For this review, take the finished solid that the model builds, in its own axes (mm). A direction names the side the tool comes from. Give positions to 0.01 mm unless a question says otherwise; leave off trailing zeros. Write item = value, one per line.
```python
from build123d import *

# Parameters (mm, degrees)
SKETCH1_R                 = 63.5
EXTRUDE1_DEPTH            = 6.35
SKETCH2_R                 = 58.7375
SKETCH2_R_2               = 52.3875
EXTRUDE2_DEPTH            = 12.7
SKETCH3_W                 = 1.5875
SKETCH3_H                 = 2.38125
CHAMFER1_SIZE             = 0.5
EXTRUDE3_DEPTH            = 6.35
F_6_CLEARANCE_HOLE1_D     = 3.7973
F_6_CLEARANCE_HOLE1_DEPTH = 330.2
F_6_CLEARANCE_HOLE1_TIP   = 1.140824014
FILLET1_R                 = 6.35
F_6_CLEARANCE_HOLE2_D     = 3.7973
F_6_CLEARANCE_HOLE2_DEPTH = 25.4
F_6_CLEARANCE_HOLE2_TIP   = 1.140824014
SKETCH8_R                 = 52.3875
CUT_EXTRUDE1_DEPTH        = 3.175


with BuildPart() as part:
    # Sketch1 → Extrude1 (new body)
    with BuildSketch(Plane(origin=(0, 0, 0), x_dir=(1, 0, 0), z_dir=(0, 1, 0))):
        Circle(SKETCH1_R)
    extrude(amount=EXTRUDE1_DEPTH)

    # Sketch2 → Extrude2 (add)
    with BuildSketch(Plane(origin=(0, 6.35, 0), x_dir=(-1, 0, 0), z_dir=(0, 1, 0))):
        Circle(SKETCH2_R)
        Circle(SKETCH2_R_2, mode=Mode.SUBTRACT)
    extrude(amount=EXTRUDE2_DEPTH)

    # Sketch3 → Cut-Revolve1 (revolve, cut)
    with BuildSketch(Plane(origin=(0, 0, 0), x_dir=(0, 0, -1), z_dir=(1, 0, 0))):
        with Locations((-57.94375, 15.656558664)):
            Rectangle(SKETCH3_W, SKETCH3_H)
        with Locations((-57.94375, 10.842416167)):
            Rectangle(SKETCH3_W, SKETCH3_H)
    revolve(axis=Axis((0, 0, 0), (0, 1, 0)), mode=Mode.SUBTRACT)

    # Chamfer1
    chamfer1_edges = [part.edges().sort_by_distance(p)[0] for p in [
        (58.7375, 16.847183664, 0),
        (58.7375, 14.465933664, 0),
        (58.7375, 12.033041167, 0),
        (58.7375, 9.651791167, 0),
        (58.7375, 19.05, 0),
        (52.3875, 19.05, 0),
    ]]
    chamfer(chamfer1_edges, length=CHAMFER1_SIZE)

    # Sketch5 → Extrude3 (add)
    with BuildSketch(Plane.XZ):
        with BuildLine():
            Line((-69.85, 9.525), (69.85, 9.525))
            ThreePointArc((69.85, 9.525), (74.340128061, 7.665128061), (76.2, 3.175))
            Line((76.2, 3.175), (76.2, -3.175))
            ThreePointArc((76.2, -3.175), (74.340128061, -7.665128061), (69.85, -9.525))
            Line((69.85, -9.525), (-69.85, -9.525))
            ThreePointArc((-69.85, -9.525), (-74.340128061, -7.665128061), (-76.2, -3.175))
            Line((-76.2, -3.175), (-76.2, 3.175))
            ThreePointArc((-76.2, 3.175), (-74.340128061, 7.665128061), (-69.85, 9.525))
        make_face()
    extrude(amount=-EXTRUDE3_DEPTH)

    # #6 Clearance Hole1
    with Locations(Plane(origin=(-69.85, 0, 0), x_dir=(0, 0, -1), z_dir=(0, -1, 0))):
        with Locations((0, 0), (0, 139.7)):
            Hole(F_6_CLEARANCE_HOLE1_D / 2, depth=F_6_CLEARANCE_HOLE1_DEPTH)
            with Locations((0, 0, -(F_6_CLEARANCE_HOLE1_DEPTH + F_6_CLEARANCE_HOLE1_TIP / 2))):  # 118° drill point
                Cone(0, F_6_CLEARANCE_HOLE1_D / 2, F_6_CLEARANCE_HOLE1_TIP, mode=Mode.SUBTRACT)

    # Fillet1
    fillet1_edges = [part.edges().sort_by_distance(p)[0] for p in [
        (62.781560788, 3.175, -9.525),
        (-62.781560788, 3.175, -9.525),
        (-62.781560788, 3.175, 9.525),
        (62.781560788, 3.175, 9.525),
    ]]
    fillet(fillet1_edges, radius=FILLET1_R)

    # #6 Clearance Hole2
    with Locations(Plane(origin=(25.4, 0, 19.05), x_dir=(0, 0, -1), z_dir=(0, -1, 0))):
        with Locations((0, 0), (-19.05, 0), (-19.05, -50.8), (0, -50.8)):
            Hole(F_6_CLEARANCE_HOLE2_D / 2, depth=F_6_CLEARANCE_HOLE2_DEPTH)
            with Locations((0, 0, -(F_6_CLEARANCE_HOLE2_DEPTH + F_6_CLEARANCE_HOLE2_TIP / 2))):  # 118° drill point
                Cone(0, F_6_CLEARANCE_HOLE2_D / 2, F_6_CLEARANCE_HOLE2_TIP, mode=Mode.SUBTRACT)

    # Sketch8 → Cut-Extrude1 (cut)
    with BuildSketch(Plane(origin=(0, 6.35, 0), x_dir=(-1, 0, 0), z_dir=(0, 1, 0))):
        Circle(SKETCH8_R)
    extrude(amount=-CUT_EXTRUDE1_DEPTH, mode=Mode.SUBTRACT)


solid = part.part
```
(1) To check wall thickness, follow probe 1 along X at (y, z) = (3.25, 0); probe 2 along X at (y, z) = (3, 0); probe 3 along Z at (x, y) = (69.85, 1.75) (3 decimals). State the ranges of each line that lie inside material, in increasing order.
Answers below:
probe_1 = -76.2 to -71.75, -67.95 to -52.39, 52.39 to 67.95, 71.75 to 76.2
probe_2 = -76.2 to -71.75, -67.95 to 67.95, 71.75 to 76.2
probe_3 = -9.525 to -1.899, 1.899 to 9.525
(2) Tool access review of faces 1 (the face through (2.513, 15.673, -57.095)), 2 (the face through (46.612, 13.239, -35.741)), 3 (the face through (-74.389, 3.131, 7.615)): name each direction out of +Z, -Z, +X, -X, +Y, -Y from which nothing blocks a thin tool from reaching the whole face with its end or side.
Answers below:
face_1 = none
face_2 = +Y
face_3 = +Z, -X, +Y, -Y
(3) Take a section at A-A (x = -25.4). Count the separate pieces of the cut face and the enclosed holes in it, plus the area to 3 significant figures.
Answers below:
separate_pieces = 3
enclosed_holes = 0
area = 587 mm^2
(4) For pin 1 (0.5 mm diameter, centred on x = -69, y = 2, fed in from +Z) (3 decimals); pin 2 (1.5 mm diameter, centred on y = 15, z = -39.5, fed in from -X); pin 3 (4 mm diameter, centred on x = -26.5, y = 12, fed in from -Z), all flat-tipped, find the tip position at first contact; note any pin that passes through.
Answers below:
pin_1 = 9.525
pin_2 = -43.3
pin_3 = -53.35
(5) The part is to be moulded in two halves that separate along Y. For faces 4 (the face through (-39, 9.652, 43)), 5 (the face through (-56, 6.35, -19)), 6 (the face through (64.029, 3.131, -10.938)), say which applies: released by +Y, released by -Y, zero draft, split by the parting line, or undercut.
Answers below:
face_4 = undercut
face_5 = released by +Y
face_6 = zero draft
